Autodesk Inventor part; units mm, degrees
ref_plane "YZ Plane" through (0, 0, 0) normal (1, 0, 0) x (0, 1, 0)
ref_plane "XZ Plane" through (0, 0, 0) normal (0, 1, 0) x (-1, 0, 0)
ref_plane "XY Plane" through (0, 0, 0) normal (0, 0, 1) x (1, 0, 0)
sketch "Náčrt2" plane through (-5.5, 0.074, 0) normal (0, 0, 1) x (1, 0, 0)
  line L0 (5.5, 7.926) -> (16.5, 7.926)
  circle A0 centre (13.5, 4.926) radius 1.5
  line L1 (16.5, 7.926) -> (16.5, 1.926)
  line L2 (16.5, 1.926) -> (-5.5, 1.926)
  line L3 (5.5, 7.926) -> (-5.5, 7.926)
  circle A1 centre (-2.5, 4.926) radius 1.5
  line L4 (-5.5, 7.926) -> (-5.5, 1.926)
  line L5 (-5.5, 7.926) -> (-25.5, 0.6466)
  line L6 (-5.5, 1.926) -> (-23.5716, -4.6515)
  line L7 (-23.5716, -4.6515) -> (-25.5, 0.6466)
  point P0 (5.5, -0.074)
  point P1 (5.5, -0.074)
  dimension "d2" = 3
  dimension "d5" = 3
  dimension "d4" = 8
  dimension "d3" = 5
  dimension "d1" = 3
  dimension "d0" = 3
  dimension "d11" = 3
  dimension "d22" = 20
  dimension "d23" = 20
  dimension "d39" = 3
  dimension "d40" = 22
  dimension "d41" = 3
extrude "Vysunutí1" add sketch "Náčrt2" along normal blind 12
fillet "Zaoblení2" radius 3 2 edges at (11, 2, 6) (11, 8, 6)
fillet "Zaoblení3" radius 10 2 edges at (-11, 2, 6) (-11, 8, 6)
fillet "Zaoblení4" radius 3 1 edges at (-29.0716, -4.5775, 6)
sketch "Náčrt3" plane through (-31, 0.7206, 12) normal (-0.3420201, 0.9396926, 0) x (0.9396926, 0.3420201, 0)
  line L0 (19.5203, 12) -> (0, 12)
  line L1 (0, 12) -> (0, 0)
  point P0 (28.884, 12)
  point P1 (16, 6)
  point P2 (6.5, 6)
  dimension "d27" = 6
  dimension "d28" = 6
  dimension "d29" = 9.5
  dimension "d30" = 16
hole "Díra2" at (-15.9649, 6.1929, 6) at (-24.892, 2.9437, 6) direction (0.3420201, -0.9396926, 0) diameter 2.9 end through all
properties part number "vrch" material "ABS plast"
Can you work these out from the model? Positions are in its coordinate system, mm. Coordinates: 2 decimals unless noted, no trailing zeros. Order: outer loops, then holes, each group sorted by start corner. A loop starts at its lowest first (then second) coordinate and runs counter-clockwise, first axis right, second up.
1. Thinking about a two-plate mould opening in Y: for faces 1 (the face through (-21.7, 4.105, 5.916)), 2 (the face through (-24.324, 0.109, 7.383)), 3 (the face through (0, 2, 6)), which applies, +Y half, -Y half, draft (parallel to the pull), parting line (faces both ways), or undercut?
2. I need wall thicknesses on line 1 (Y direction, x = -8, z = 6); line 2 (Y direction, x = 4, z = 3); line 3 (Z direction, x = -14, y = 1.75). Which ranges of each line are inside material? Lowest first, please.
3. If we section it at A-A (x = -8): Please give me the cut outline in (y, z).
4. If we section it at B-B (z = 6.5): Give the number of separate pieces and of enclosed holes in the cut face, then the cut area to 3 significant figures.
5. I'm going to push flat-ended pins straight in: pin 1 (3.5 mm diameter, centred on x = 8, y = 5, fed in from -Z); pin 2 (3.5 mm diameter, centred on x = -3, z = 6, fed in from -Y); pin 3 (3 mm diameter, centred on x = -19.5, z = 4, fed in from +Y). Where does each tip first touch, or does it pass through?
Entries:
1. face 1: +Y half
1. face 2: undercut
1. face 3: -Y half
2. line 1: y = 2 to 3.5, 6.5 to 8
2. line 2: y = 2 to 8
2. line 3: z = 0 to 4.59, 7.41 to 12
3. outline: (2, 0) - (3.5, 0) - (3.5, 12) - (2, 12) - close; (6.5, 0) - (8, 0) - (8, 12) - (6.5, 12) - close
4. separate pieces: 3
4. enclosed holes: 2
4. area: 196 mm2
5. pin 1: stops at z = 0
5. pin 2: stops at y = 2
5. pin 3: stops at y = 5.45
